Model file for the job. Use its own axes, mm. Face numbers are marked on the shaded views. Coordinates: 2 decimals unless noted, no trailing zeros. Order: outer loops, then holes, each group sorted by start corner. A loop starts at its lowest first (then second) coordinate and runs counter-clockwise, first axis right, second up. Notation, with made-up numbers: M 82,43.25 L 126,43.25 A10 cw 126,50.25 Z; hole C -25,45 d3. An arc over 180 degrees is marked long. Return JSON: item names as keys, results as strings.
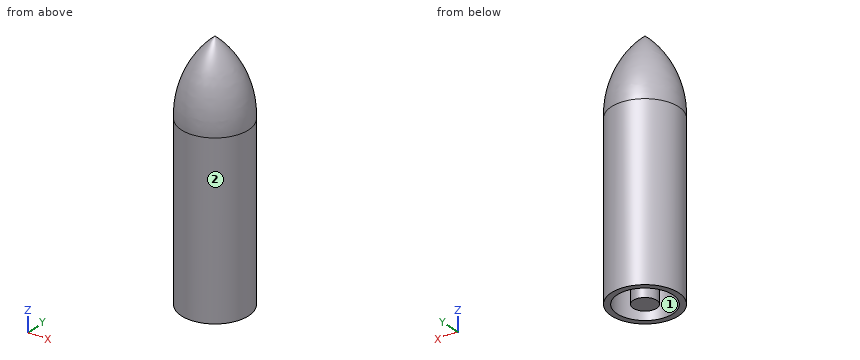
```python
from build123d import *


with BuildPart() as f1:
    # F0 (on Right) → F1 (revolve)
    with BuildSketch(Plane.YZ):
        with BuildLine():
            Line((0, 1625.6), (0, 0))
            Line((0, 0), (101.6, 0))
            Line((101.6, 0), (101.6, 240.015262))
            ThreePointArc((101.6, 240.015262), (116.364586, 271.734327), (150.140911, 280.858576))
            ThreePointArc((150.140911, 280.858576), (202.921417, 283.418504), (228.6, 329.602327))
            Line((228.6, 329.602327), (228.6, 1269.53539))
            ThreePointArc((228.6, 1269.53539), (166.531015, 1481.100963), (0, 1625.6))
        make_face()
    revolve(axis=Axis((0, 0, 812.8), (0, 0, 1)))

    # F2 (on Right) → F3 (revolve)
    with BuildSketch(Plane.YZ):
        with BuildLine():
            Line((0, 2137.444043), (0, 1588.585455))
            Line((0, 1588.585455), (241.3, 1258.340002))
            Line((241.3, 1258.340002), (241.3, 0))
            Line((241.3, 0), (292.1, 0))
            Line((292.1, 0), (292.1, 1481.604533))
            ThreePointArc((292.1, 1481.604533), (220.424698, 1842.64954), (0, 2137.444043))
        make_face()
    revolve(axis=Axis((0, 0, 1068.722021), (0, 0, 1)))


solid = f1.part
```
Item 1: Pull direction X, two halves, no side cores. Call the marked faces 1 and 2: +X half, -X half, draft (parallel to the pull), parting line (faces both ways), or undercut.
Check result:
{"face 1": "undercut", "face 2": "parting line"}
Item 2: Saw through at A-A (z = 434). Write the cut outline in (x, y).
Check result:
{"outline": "C 0,0 d584.2; C 0,0 d457.2; hole C 0,0 d482.6"}
Item 3: Drop flat-ended pins along their axis: pin 1 Ø8 at (x, z) = (15.5, 800.5) entering from -Y; pin 2 Ø5 at (y, z) = (83.5, 1321.5) entering from -X; pin 3 Ø6 at (y, z) = (-161, 1231) entering from -X. Give the stop position or say it passes through.
Check result:
{"pin 1": "stops at y = -291.87", "pin 2": "stops at x = -280.64", "pin 3": "stops at x = -245.68"}
Item 4: Saw through at B-B (z = 129.5). Write the cut outline in (x, y).
Check result:
{"outline": "C 0,0 d584.2; C 0,0 d203.2; hole C 0,0 d482.6"}
Item 5: Wall check: line 1 (Y direction, x = 0, z = 968); line 2 (X direction, y = 20, z = 806). Give the ranges that are in metal, low to high.
Check result:
{"line 1": "y = -292.1 to -241.3, -228.6 to 228.6, 241.3 to 292.1", "line 2": "x = -291.41 to -240.47, -227.72 to 227.72, 240.47 to 291.41"}
Item 6: Saw through at C-C (z = 1375.5). Write the cut outline in (x, y).
Check result:
{"outline": "C 0,0 d584.2"}
